Autodesk Inventor part; units mm, degrees
ref_plane "YZ Plane" through (0, 0, 0) normal (1, 0, 0) x (0, 1, 0)
ref_plane "XZ Plane" through (0, 0, 0) normal (0, 1, 0) x (-1, 0, 0)
ref_plane "XY Plane" through (0, 0, 0) normal (0, 0, 1) x (1, 0, 0)
sketch "Sketch1" plane through (0, 0, 0) normal (0, 1, 0) x (-1, 0, 0)
  circle A0 centre (0, 0) radius 25
  circle A1 centre (0, 0) radius 30
  circle A2 centre (0, 0) radius 17.5
  line L0 (0, 0) -> (25, 0) construction
  circle A3 centre (17.6777, -17.6777) radius 2
  circle A4 centre (17.6777, 17.6777) radius 2
  circle A5 centre (-17.6777, 17.6777) radius 2
  circle A6 centre (-17.6777, -17.6777) radius 2
  point P0 (0, -27.5)
  point P1 (0, -27.5)
  point P2 (27.5, 0)
  point P3 (-27.5, 0)
  point P4 (0, 27.5)
  dimension "d0" = 50
  dimension "d1" = 60
  dimension "d17" = 27.5
  dimension "d18" = 27.5
  dimension "d19" = 27.5
  dimension "d20" = 27.5
  dimension "d28" = 35
  dimension "d30" = 4
  dimension "d33" = 360
extrude "Extrusion1" add sketch "Sketch1" along normal blind 5 contours A0 A4 | A3 A0 | A0 A5 | A6 A0 | A1 picked at (18.1752, 18.1125) picked at (18.1752, -18.1125) picked at (-18.083, 18.1995) picked at (-18.083, -18.1995)
extrude "Extrusion2" add sketch "Sketch1" against normal blind 5 contours A0 A3 A6 A5 A4 | A4 A0 | A0 A4 | A3 A0 | A0 A3 | A5 A0 | A0 A5 | A6 A0 | A0 A6 | A1
hole "Hole2" at (0, 0, -27.5) at (-27.5, 0, 0) at (27.5, 0, 0) at (0, 0, 27.5) direction (0, 1, 0) diameter 2.45 end through all both
sketch "Sketch2" plane through (0, -5, 0) normal (0, -1, 0) x (1, 0, 0)
  circle A0 centre (0, 0) radius 22.5
  line L0 (0, 0) -> (15.9099, 15.9099)
  line L1 (0, 0) -> (22.5, 0) construction
  circle A1 centre (15.9099, 15.9099) radius 3
  circle A2 centre (-15.9099, 15.9099) radius 3
  circle A3 centre (-15.9099, -15.9099) radius 3
  circle A4 centre (15.9099, -15.9099) radius 3
  dimension "d35" = 45
  dimension "d36" = 45
  dimension "d37" = 6
  dimension "d40" = 360
extrude "Extrusion3" cut sketch "Sketch2" against normal blind 5 contours A1 L0 A0 | A0 A1 | A4 A0 | A0 A4 | L0 A1 A0 | A3 A0 | A0 A3 | A2 A0 | A0 A2
thread "Thread1"
thread "Thread2"
thread "Thread3"
thread "Thread4"
properties part number "Placeholderjointouterring"
Input: part model. Units: mm. Frame: model coordinates. A direction names the side the tool comes from. Round coordinates to 2 decimals unless told otherwise and drop trailing zeros. Order: outer loops, then holes, each group sorted by start corner. A loop starts at its lowest first (then second) coordinate and runs counter-clockwise, first axis right, second up.
1. Pin query (flat end, axial travel): P1, Ø4, axis at y = 2, z = 17.5, coming from the -X side; P2, Ø1.5, axis at x = 12, y = 0.5, coming from the -Z side; P3, Ø3, axis at x = -20, y = -1.5, coming from the +Z side; P4, Ø1.2, axis at x = 17, z = -17, coming from the -Y side. Return the tip coordinate at first contact, or that it passes through.
The answers:
P1: stops at x = -25.69
P2: stops at z = -27.81
P3: stops at z = 23.62
P4: passes through
2. Cut plane C-C, the plane z = -8.5. Output: boundary loops of the cut face in (x, y), then the cut area to 3 significant figures.
The answers:
outline: (-28.77, -5) - (-15.3, -5) - (-15.3, 0) - (-23.51, 0) - (-23.51, 5) - (-28.77, 5) - close; (15.3, -5) - (28.77, -5) - (28.77, 5) - (23.51, 5) - (23.51, 0) - (15.3, 0) - close
area: 187 mm2
3. Cut plane D-D, the plane y = -3.5. State how many separate pieces and enclosed holes the cut face has, then the cut area to 3 significant figures.
The answers:
separate pieces: 1
enclosed holes: 9
area: 1,730 mm2
4. Cut plane B-B, the plane x = 0. Output: boundary loops of the cut face in (y, z) (3 decimals), then the cut area to 3 significant figures.
The answers:
outline: (-5, -30) - (5, -30) - (5, -28.725) - (-5, -28.725) - close; (-5, -26.275) - (5, -26.275) - (5, -25) - (0, -25) - (0, -17.5) - (-5, -17.5) - close; (-5, 17.5) - (0, 17.5) - (0, 25) - (5, 25) - (5, 26.275) - (-5, 26.275) - close; (-5, 28.725) - (5, 28.725) - (5, 30) - (-5, 30) - close
area: 126 mm2
5. Mould query, pull axis X, two halves, no side actions, for faces 4 (the face through (5, 5, 25)), 5 (the face through (29.97, -0.07, -1.32)), 6 (the face through (17.8, 0, 17.8)). Classes: released by +X, released by -X, zero draft, split by the parting line, or undercut.
The answers:
face 4: zero draft
face 5: split by the parting line
face 6: undercut
6. Material intervals for line 1 (Z direction, x = 0, y = 1.05) (3 decimals); line 2 (Y direction, x = -6, z = 23); line 3 (Z direction, x = -5, y = 0.25), sorted ascending.
The answers:
line 1: z = -30 to -28.725, -26.275 to -25, 25 to 26.275, 28.725 to 30
line 2: y = -5 to 0
line 3: z = -29.58 to -24.49, 24.49 to 29.58
7. Cut plane A-A, the plane z = 0. Output: boundary loops of the cut face in (x, y) (3 decimals).
The answers:
outline: (-30, -5) - (-28.725, -5) - (-28.725, 5) - (-30, 5) - close; (-26.275, -5) - (-17.5, -5) - (-17.5, 0) - (-25, 0) - (-25, 5) - (-26.275, 5) - close; (17.5, -5) - (26.275, -5) - (26.275, 5) - (25, 5) - (25, 0) - (17.5, 0) - close; (28.725, -5) - (30, -5) - (30, 5) - (28.725, 5) - close
8. Set-up query: faces 1 (the face through (-28.715, 0.07, 0.159)), 2 (the face through (15.26, -2.54, 12.98)), 3 (the face through (-5, 0, 17)). Return all of +Z, -Z, +X, -X, +Y, -Y with unobstructed straight access to the full face (end or side cutting, diameter ignored); none if empty.
The answers:
face 1: +Y, -Y
face 2: -Y
face 3: +Y
